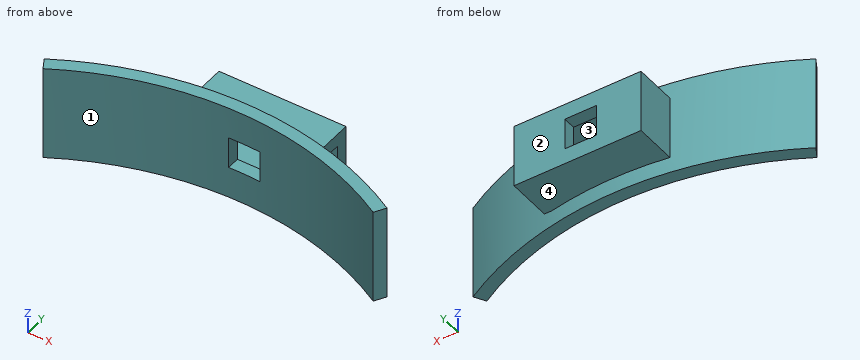
```python
from build123d import *

# Parameters (mm, degrees)
BOX002_W                    = 20
BOX002_H                    = 4
BOX002_DEPTH                = 6
BOX_W                       = 5
BOX_H                       = 20
BOX_DEPTH                   = 5
BOX001_W                    = 20
BOX001_H                    = 7
BOX001_DEPTH                = 10
CYLINDER001_W               = 52
CYLINDER001_H               = 15
CYLINDER001_ANGLE           = 60
CYLINDER001_PLACEMENT_ANGLE = 60
CYLINDER_W                  = 54
CYLINDER_H                  = 15
CYLINDER_ANGLE              = 60
CYLINDER_PLACEMENT_ANGLE    = 60


with BuildPart() as slot:
    # Box002 → Box002 (new body)
    with BuildSketch(Plane(origin=(2, 45, 4.5), x_dir=(1, 0, 0), z_dir=(0, 0, 1))):
        with Locations((10, 2)):
            Rectangle(BOX002_W, BOX002_H)
    extrude(amount=BOX002_DEPTH)


with BuildPart() as pin_opening:
    # Box → Box (new body)
    with BuildSketch(Plane(origin=(7, 42, 5), x_dir=(1, 0, 0), z_dir=(0, 0, 1))):
        with Locations((2.5, 10)):
            Rectangle(BOX_W, BOX_H)
    extrude(amount=BOX_DEPTH)


with BuildPart() as latch:
    # Box001 → Box001 (new body)
    with BuildSketch(Plane(origin=(0, 44, 2.5), x_dir=(1, 0, 0), z_dir=(0, 0, 1))):
        with Locations((10, 3.5)):
            Rectangle(BOX001_W, BOX001_H)
    extrude(amount=BOX001_DEPTH)


with BuildPart() as bottle_wall001:
    # Cylinder001 → Cylinder001 (revolve)
    with BuildSketch(Plane.XZ):
        with Locations((26, 7.5)):
            Rectangle(CYLINDER001_W, CYLINDER001_H)
    revolve(axis=Axis((0, 0, 0), (0, 0, 1)), revolution_arc=CYLINDER001_ANGLE)


with BuildPart() as bottle_wall001_1:
    # Cylinder001 placement: moved
    add(bottle_wall001.part.moved(Location((8.5, -7, 0))).rotate(Axis((8.5, -7, 0), (0, 0, 1)), CYLINDER001_PLACEMENT_ANGLE))


with BuildPart() as cut002:
    # Cylinder → Cylinder (revolve)
    with BuildSketch(Plane.XZ):
        with Locations((27, 7.5)):
            Rectangle(CYLINDER_W, CYLINDER_H)
    revolve(axis=Axis((0, 0, 0), (0, 0, 1)), revolution_arc=CYLINDER_ANGLE)


with BuildPart() as cut002_1:
    # Cylinder placement: moved
    add(cut002.part.moved(Location((8.5, -7, 0))).rotate(Axis((8.5, -7, 0), (0, 0, 1)), CYLINDER_PLACEMENT_ANGLE))

    # Cut: cut bottle_wall001
    add(bottle_wall001_1.part, mode=Mode.SUBTRACT)


with BuildPart() as cut002_2:
    # Cut placement: moved
    add(cut002_1.part.moved(Location((0, -2, 0))))

    # Fusion: union latch
    add(latch.part)

    # Fusion001: union latch
    add(latch.part)

    # Cut001: cut pin_opening
    add(pin_opening.part, mode=Mode.SUBTRACT)

    # Cut002: cut slot
    add(slot.part, mode=Mode.SUBTRACT)


solid = cut002_2.part
```
Here's how the part is built. I have some questions about the finished solid (model axes, mm). Face numbers are marked on the shaded views. Coordinates: 2 decimals unless noted, no trailing zeros. Write each loop counter-clockwise with the first axis right and the second up, starting at its lowest first coordinate (ties: lowest second). Pieces come first, ordered by that corner, then holes. Notation, with made-up numbers: (17, 72.25) -> (76, 72.25) arc R38 ccw to (76, 111.25) -> close; hole circle Ø5 at (75, -7). An arc over 180 degrees is marked (long way). Use a Markdown table: item, result. Add a question column.
(1) Please list where these lines run through material, in increasing order: line 1 (Z direction, x = 10.5, y = 45.5); line 2 (X direction, y = 47.5, z = 8.5); line 3 (Y direction, x = 32, z = 2.25).
(2) If we section it at D-D, the plane z = 4: Write out the boundary of the cut face in (x, y), and give its area (3 significant figures).
(3) We'd pull the mould along Y, two halves only. Please class the marked faces 1, 2, 3 and 4: +Y half, -Y half, draft (parallel to the pull), parting line (faces both ways), or undercut.
(4) If we section it at B-B, the plane y = 41: Write out the boundary of the cut face in (x, z), and give its area (3 significant figures).
(5) I'm going to push flat-ended pins straight in: P1, Ø3, axis at x = 0.5, z = 11, coming from the -Y side; P2, Ø5, axis at x = 19.5, y = 47.5, coming from the +Z side; P3, Ø0.6, axis at x = 19.5, z = 6, coming from the -Y side. Where does each tip first touch, or does it pass through?
(6) If we section it at A-A, the plane z = 6.75: Write out the boundary of the cut face in (x, y), and give its area (3 significant figures).
(7) If we section it at C-C, the plane x = 14.5: Write out the boundary of the cut face in (y, z).
Outcome:
| question | item | result |
|---|---|---|
| 1 | line 1 | z = 2.5 to 4.5, 10.5 to 12.5 |
| 1 | line 2 | x = 0 to 2 |
| 1 | line 3 | y = 37.39 to 39.62 |
| 2 | outline | (-18.5, 37.77) -> (-17.5, 36.03) arc R52 cw to (34.5, 36.03) -> (35.5, 37.77) arc R54 ccw to (18.84, 44) -> (20, 44) -> (20, 51) -> (0, 51) -> (0, 44.33) arc R54 ccw to start |
| 2 | area | 237 mm^2 |
| 3 | face 1 | -Y half |
| 3 | face 2 | +Y half |
| 3 | face 3 | undercut |
| 3 | face 4 | draft |
| 4 | outline | (-11.9, 0) -> (-5.78, 0) -> (-5.78, 15) -> (-11.9, 15) -> close; (22.78, 0) -> (28.9, 0) -> (28.9, 15) -> (22.78, 15) -> close |
| 4 | area | 183 mm^2 |
| 5 | P1 | stops at y = 42.12 |
| 5 | P2 | stops at z = 12.5 |
| 5 | P3 | stops at y = 41.76 |
| 6 | outline | (-18.5, 37.77) -> (-17.5, 36.03) arc R52 cw to (7, 42.98) -> (7, 45) -> (2, 45) -> (2, 49) -> (7, 49) -> (7, 51) -> (0, 51) -> (0, 44.33) arc R54 ccw to start; (12, 42.88) arc R52 cw to (34.5, 36.03) -> (35.5, 37.77) arc R54 ccw to (18.84, 44) -> (20, 44) -> (20, 45) -> (12, 45) -> close; (12, 49) -> (20, 49) -> (20, 51) -> (12, 51) -> close |
| 6 | area | 145 mm^2 |
| 7 | outline | (42.65, 0) -> (44.67, 0) -> (44.67, 2.5) -> (51, 2.5) -> (51, 12.5) -> (44.67, 12.5) -> (44.67, 15) -> (42.65, 15) -> close; hole (45, 4.5) -> (49, 4.5) -> (49, 10.5) -> (45, 10.5) -> close |
